```python
from build123d import *

# Parameters (mm, degrees)
SKETCH1_W                                        = 19.05
SKETCH1_H                                        = 450.85
BOSS_EXTRUDE1_DEPTH                              = 66.675
FILLET4_R                                        = 38.1
CUT_EXTRUDE1_REACH                               = 458.151
BOSS_EXTRUDE2_DEPTH                              = 19.05
BOSS_EXTRUDE3_DEPTH                              = 19.05
F_1_4_0_25_DIAMETER_HOLE1_D                      = 6.35
F_10_CLEARANCE_HOLE_WITH_1_0_X_25_CB_D           = 5.6134
F_10_CLEARANCE_HOLE_WITH_1_0_X_25_CB_CBORE_D     = 12.7
F_10_CLEARANCE_HOLE_WITH_1_0_X_25_CB_CBORE_DEPTH = 6.35
F_1_2_0_5_DIAMETER_SLOT1_D                       = 12.7


with BuildPart() as part:
    # Sketch1 → Boss-Extrude1 (new body)
    with BuildSketch(Plane.XY):
        with Locations((-218.563766336, -225.425)):
            Rectangle(SKETCH1_W, SKETCH1_H)
    extrude(amount=BOSS_EXTRUDE1_DEPTH)

    # Fillet4
    fillet4_edges = [part.edges().sort_by_distance(p)[0] for p in [
        (-218.563766336, -450.85, 66.675),
    ]]
    fillet(fillet4_edges, radius=FILLET4_R)

    # Sketch4 → Cut-Extrude1 (cut, up to next)
    with BuildSketch(Plane.ZY.offset(228.088766336), mode=Mode.PRIVATE) as cut_extrude1_sk1:
        with BuildLine():
            Line((66.675, 0), (66.675, -412.75))
            ThreePointArc((66.675, -412.75), (55.515768363, -439.690768363), (28.575, -450.85))
            Line((28.575, -450.85), (28.575, -444.5))
            ThreePointArc((28.575, -444.5), (51.025640303, -435.200640303), (60.325, -412.75))
            Line((60.325, -412.75), (60.325, 0))
            Line((60.325, 0), (66.675, 0))
        make_face()
    cut_extrude1_tool1 = extrude(cut_extrude1_sk1.sketch, amount=-CUT_EXTRUDE1_REACH, mode=Mode.PRIVATE) & part.part
    add(cut_extrude1_tool1.solids().sort_by_distance((-228.088766, -233.202612, 62.01827))[0], mode=Mode.SUBTRACT)

    # Sketch7 → Boss-Extrude2 (add, through all)
    with BuildSketch(Plane.ZY.offset(228.088766336)):
        Polygon((0, 0), (60.325, 0), (60.325, 34.844553242), (0, 20.824633003), align=None)
    extrude(amount=-BOSS_EXTRUDE2_DEPTH)

    # Sketch8 → Boss-Extrude3 (add, through all)
    with BuildSketch(Plane.ZY.offset(228.088766336)):
        Polygon((60.325, 34.844553242), (83.828599938, 40.306941911), (93.196193981, 0), (60.325, 0), align=None)
    extrude(amount=-BOSS_EXTRUDE3_DEPTH)

    # 1/4 (0.25) Diameter Hole1 (through all)
    with Locations(Plane.ZY.offset(228.088766336)):
        with Locations((28.575, -444.5), (60.325, 0)):
            Hole(F_1_4_0_25_DIAMETER_HOLE1_D / 2)

    # #10 Clearance Hole with 1.0 x .25 CB (through all)
    with Locations(Plane.ZY.offset(228.088766336)):
        with Locations((37.58012522, -0.660555349)):
            CounterBoreHole(F_10_CLEARANCE_HOLE_WITH_1_0_X_25_CB_D / 2, F_10_CLEARANCE_HOLE_WITH_1_0_X_25_CB_CBORE_D / 2, F_10_CLEARANCE_HOLE_WITH_1_0_X_25_CB_CBORE_DEPTH)

    # 1/2 (0.5) Diameter Slot1 (through all)
    with Locations(Plane.ZY.offset(228.088766336)):
        with Locations((14.175520603, -6.646762989)):
            Hole(F_1_2_0_5_DIAMETER_SLOT1_D / 2)


solid = part.part
```
Model file for the job. Use its own axes, mm. A direction names the side the tool comes from. Give positions to 0.01 mm unless a question says otherwise; leave off trailing zeros. Write each loop counter-clockwise with the first axis right and the second up, starting at its lowest first coordinate (ties: lowest second). Pieces come first, ordered by that corner, then holes. Notation, with made-up numbers: (40.25, 48.25) - (81.25, 48.25) arc R33 cw to (81.25, 77.25) - close; hole circle Ø5 at (83.5, 19). An arc over 180 degrees is marked (long way). One line per question, with ' | ' between items. Start each with the question number.
(1) 3-axis set-ups, long thin cutter, end or side, ignore diameter. For faces 4 (the face through (-224.96, -4.52, 32.54)), 5 (the face through (-219, -212, 0)), 6 (the face through (-219, 0, 79)): which of +Z, -Z, +X, -X, +Y, -Y reach the whole face in a straight line?
(2) Slice it at C-C on z = 74. Write the cut outline in (x, y).
(3) Wall check: line 1 along Z through (x, y) = (-212.5, -363) (3 decimals); line 2 along Y through (x, z) = (-222.5, 18.5); line 3 along Y through (x, z) = (-224.5, 12.5). Give the ranges that are in metal, low to high. Write a range as from..to.
(4) Slice it at B-B on y = -97. Write the cut outline in (x, z) (3 decimals), plus the area to 3 significant figures.
(5) Pin check, flat tips, straight feed: P1, Ø8, axis at x = -216, y = -378.5, coming from the -Z side; P2, Ø6, axis at x = -211.5, z = 58, coming from the +Y side; P3, Ø3.5, axis at y = -0.66, z = 37.58, coming from the -X side; P4, Ø1, axis at x = -226, z = 47.5, coming from the -Y side. Stop position of each tip, or through.
(6) Slice it at A-A on x = -215.5. Write the cut outline in (y, z) (3 decimals).
(7) Two-plate mould, pull along Y, no slides. Class faces 1 (the face through (-219, -450.85, 14)), 2 (the face through (-209.039, -202, 37)), 3 (the face through (-218.43, -12.28, 11.245)): +Y half, -Y half, draft (parallel to the pull), parting line (faces both ways), or undercut.
Results below:
1) face 4: -X | face 5: -Z, +X, -X, +Y, -Y | face 6: +Z, +X, -X, -Y
2) outline: (-228.09, 0) - (-209.04, 0) - (-209.04, 38.02) - (-228.09, 38.02) - close
3) line 1: 0..60.325 | line 2: -450.85..-11.3, -2..25.12 | line 3: -450.85..-12.77, -0.52..23.73
4) outline: (-228.089, 0) - (-209.039, 0) - (-209.039, 60.325) - (-228.089, 60.325) - close | area: 1,150 mm^2
5) P1: z = 0 | P2: y = 35 | P3: through | P4: y = -438.61
6) outline: (-450.85, 0) - (20.825, 0) - (40.307, 83.829) - (0, 93.196) - (0, 63.5) arc R3.175 cw (long way) to (-3.175, 60.325) - (-412.75, 60.325) arc R31.75 ccw to (-444.341, 31.746) arc R3.175 cw (long way) to (-447.675, 28.575) - (-450.85, 28.575) - close; hole circle Ø12.7 at (-6.647, 14.176); hole circle Ø5.613 at (-0.661, 37.58)
7) face 1: -Y half | face 2: draft | face 3: undercut
